Check sheet for the modelled part. Datum: model origin and axes. Units: mm. A direction names the side the tool comes from. Coordinates: 2 decimals unless noted, no trailing zeros. Loops run counter-clockwise (first coordinate to the right, second up) from the corner with the lowest first, then second, coordinate; pieces in that order, holes last. Notation, with made-up numbers: (50.5, 83) -> (104.5, 83) arc R23 ccw to (104.5, 106) -> close; hole circle Ø10 at (-18, -15.75). An arc over 180 degrees is marked (long way). Use one line per item in the form item = value.
from build123d import *

# Parameters (mm, degrees)
F2_SIZE        = 1
F4_D           = 6.6
F4_CSINK_D     = 13.44
F4_CSINK_ANGLE = 90
F6_D           = 8.4
F6_CBORE_D     = 14.25
F6_CBORE_DEPTH = 8


with BuildPart() as f1:
    # F0 (on Front) → F1 (revolve)
    with BuildSketch(Plane.XZ):
        Polygon((0, 10), (0, 0), (31.6, 0), (31.6, -7), (35.6, -7), (35.6, 10), align=None)
        Polygon((0, 22), (0, 10), (35.6, 10), (54, 10), (54, 22), align=None)
    revolve(axis=Axis((0, 0, 5), (0, 0, -1)))

    # F2
    f2_edges = [f1.edges().sort_by_distance(p)[0] for p in [
        (-31.6, 0, -7),
        (-35.6, 0, -7),
        (-35.6, 0, 10),
    ]]
    chamfer(f2_edges, length=F2_SIZE)

    # F4 (through all)
    with Locations(Plane.XY.offset(22)):
        with Locations((-25, 0), (25, 0), (0, -25), (0, 25)):
            CounterSinkHole(F4_D / 2, F4_CSINK_D / 2, counter_sink_angle=F4_CSINK_ANGLE)

    # F6 (through all)
    with Locations(Plane(origin=(0, 0, 10), x_dir=(1, 0, 0), z_dir=(0, 0, -1))):
        with Locations((-38.9711431703, -22.5), (38.9711431703, -22.5), (0, 45)):
            CounterBoreHole(F6_D / 2, F6_CBORE_D / 2, F6_CBORE_DEPTH)


solid = f1.part
(1) Section check A-A, the plane z = 13. Record the boundary of the cut face in (x, y) (3 decimals).
Established:
outline = circle Ø108 at (0, 0); hole circle Ø14.25 at (-38.971, 22.5); hole circle Ø6.6 at (-25, 0); hole circle Ø14.25 at (0, -45); hole circle Ø6.6 at (0, -25); hole circle Ø6.6 at (0, 25); hole circle Ø6.6 at (25, 0); hole circle Ø14.25 at (38.971, 22.5)
(2) Go/stop test with flat-tipped pins: P1, Ø5, axis at x = 35, z = -3, coming from the +Y side; P2, Ø2, axis at x = 28, z = 12.5, coming from the +Y side; P3, Ø1, axis at x = 12, z = 9, coming from the -Y side. Record where each tip stops, or that it passes through.
Established:
P1 = 14.53
P2 = 46.77
P3 = -34.08
(3) Tool access check on faces 1 (the cylindrical face through (-25.1, 19.2, -3)), 2 (the cylindrical face through (0.72, 21.78, 9.16)). Record the directions out of +Z, -Z, +X, -X, +Y, -Y that give a thin tool (end or side, any length) a straight path to the whole face; none if there is none.
Established:
face_1 = -Z
face_2 = +Z, -Z
(4) Section check D-D, the plane y = -45. Record the boundary of the cut face in (x, z) (3 decimals).
Established:
outline = (-29.85, 10) -> (-7.125, 10) -> (-7.125, 18) -> (-4.2, 18) -> (-4.2, 22) -> (-29.85, 22) -> close; (4.2, 18) -> (7.125, 18) -> (7.125, 10) -> (29.85, 10) -> (29.85, 22) -> (4.2, 22) -> close
(5) Scan lines: line 1 along Y through (x, z) = (0, 12.5) (3 decimals); line 2 along Y through (x, z) = (3, 20.5); line 3 along X through (y, z) = (22.5, 13.25). Record each from-to range of solid material in increasing order.
Established:
line_1 = -54 to -52.125, -37.875 to -28.3, -21.7 to 21.7, 28.3 to 54
line_2 = -53.92 to -47.94, -42.06 to -29.27, -20.73 to 20.73, 29.27 to 53.92
line_3 = -49.09 to -46.1, -31.85 to -2.15, 2.15 to 31.85, 46.1 to 49.09
(6) Section check B-B, the plane y = 0. Give the number of separate pieces and of enclosed holes in the cut face, plus the area to 3 significant figures.
Established:
separate_pieces = 3
enclosed_holes = 0
area = 1,750 mm²
(7) Section check C-C, the plane x = -39.5. Record the boundary of the cut face in (y, z), plus the area to 3 significant figures.
Established:
outline = (-36.82, 10) -> (15.39, 10) -> (15.39, 18) -> (18.33, 18) -> (18.33, 22) -> (-36.82, 22) -> close; (26.67, 18) -> (29.61, 18) -> (29.61, 10) -> (36.82, 10) -> (36.82, 22) -> (26.67, 22) -> close
area = 737 mm²
(8) Mould release check, pull along Y, two halves, no side actions. Record for faces 3 (the cylindrical face through (-11.706, 52.716, 16.084)), 4 (the flat face through (-1, -1, 22)), 5 (the cylindrical face through (0.72, -28.22, 9.16)): +Y half, -Y half, draft (parallel to the pull), parting line (faces both ways), or undercut.
Established:
face_3 = parting line
face_4 = draft
face_5 = undercut
